```python
from build123d import *

# Parameters (mm, degrees)
BOSS_EXTRUDE1_DEPTH = 11.35
CUT_EXTRUDE1_DEPTH  = 6.35
BOSS_EXTRUDE2_DEPTH = 47
CUT_EXTRUDE2_DEPTH  = 47


with BuildPart() as part:
    # Sketch1 → Boss-Extrude1 (new body, symmetric)
    with BuildSketch(Plane.XY):
        Polygon((0, 0), (0, 47), (-17, 47), (-47, 17), (-47, 0), align=None)
    extrude(amount=BOSS_EXTRUDE1_DEPTH, both=True)

    # Sketch2 → Cut-Extrude1 (cut, symmetric)
    with BuildSketch(Plane.XY):
        Polygon((-47, 17), (-47, 2), (-2, 2), (-2, 47), (-17, 47), align=None)
    extrude(amount=CUT_EXTRUDE1_DEPTH, both=True, mode=Mode.SUBTRACT)

    # Sketch3 → Boss-Extrude2 (add)
    with BuildSketch(Plane(origin=(0, 0, -11.35), x_dir=(-1, 0, 0), z_dir=(0, 0, -1))):
        Polygon((0, 0), (0, 2), (0, 14.7), (0, 16.7), (47, 16.7), (47, 14.7), (2, 14.7), (2, 2), (47, 2), (47, 0), align=None)
    extrude(amount=BOSS_EXTRUDE2_DEPTH)

    # Sketch4 → Cut-Extrude2 (cut)
    with BuildSketch(Plane(origin=(0, 16.7, 0), x_dir=(1, 0, 0), z_dir=(0, 1, 0))):
        Polygon((-17, 58.35), (-47, 28.35), (-47, 58.35), align=None)
    extrude(amount=-CUT_EXTRUDE2_DEPTH, mode=Mode.SUBTRACT)


solid = part.part
```
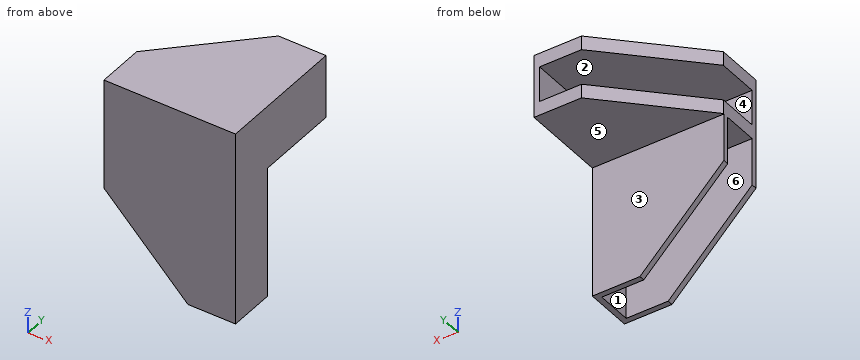
Model file for the job. Use its own axes, mm. Face numbers are marked on the shaded views. A direction names the side the tool comes from. Give positions to 0.01 mm unless a question says otherwise; leave off trailing zeros. Order: outer loops, then holes, each group sorted by start corner. A loop starts at its lowest first (then second) coordinate and runs counter-clockwise, first axis right, second up.
1) Saw through at D-D, the plane y = 6.5. Write the cut outline in (x, z), then the cut area to 3 significant figures.
2) Wall check: probe 1 along Y at (x, z) = (-7, -42); probe 2 along Z at (x, y) = (-26, 30); probe 3 along X at (y, z) = (9, -50). Give the ranges that are in metal, low to high.
3) Saw through at C-C, the plane x = -37. Write the cut outline in (y, z), then the cut area to 3 significant figures.
4) Mould opens along Z. For the marked faces 4, 5 and 6 say: +Z half, -Z half, draft (parallel to the pull), parting line (faces both ways), or undercut.
5) Pin check, flat tips, straight feed: pin 1 (22.5 mm diameter, centred on x = -17, y = 29.5, fed in from -Z); pin 2 (4 mm diameter, centred on x = -21, z = 0.5, fed in from +Y); pin 3 (2 mm diameter, centred on y = 18, z = -26, fed in from +X); pin 4 (10 mm diameter, centred on y = 7.5, z = -29.5, fed in from -X). Stop position of each tip, or through.
6) Saw through at A-A, the plane z = -20. Write the cut outline in (x, y).
7) 3-axis set-ups, long thin cutter, end or side, ignore diameter. For the marked faces 1, 2 and 3: which of +Z, -Z, +X, -X, +Y, -Y reach the whole face in a straight line?
8) Saw through at B-B, the plane y = 42. Write the cut outline in (x, z), then the cut area to 3 significant figures.
Computed:
1. outline: (-47, -11.35) - (-2, -11.35) - (-2, -58.35) - (0, -58.35) - (0, 11.35) - (-47, 11.35) - (-47, 6.35) - (-2, 6.35) - (-2, -6.35) - (-47, -6.35) - close
1. area: 589 mm2
2. probe 1: y = 0 to 2, 14.7 to 16.7
2. probe 2: z = -11.35 to -6.35, 6.35 to 11.35
2. probe 3: x = -2 to 0
3. outline: (0, -38.35) - (2, -38.35) - (2, -11.35) - (14.7, -11.35) - (14.7, -38.35) - (16.7, -38.35) - (16.7, -11.35) - (27, -11.35) - (27, -6.35) - (2, -6.35) - (2, 6.35) - (27, 6.35) - (27, 11.35) - (0, 11.35) - close
3. area: 403 mm2
4. face 4: undercut
4. face 5: -Z half
4. face 6: draft
5. pin 1: stops at z = -11.35
5. pin 2: stops at y = 2
5. pin 3: passes through
5. pin 4: stops at x = -2
6. outline: (-47, 0) - (0, 0) - (0, 16.7) - (-47, 16.7) - (-47, 14.7) - (-2, 14.7) - (-2, 2) - (-47, 2) - close
7. face 1: -Z, -X
7. face 2: -X, +Y
7. face 3: -Z, +X, -X, +Y
8. outline: (-22, -11.35) - (0, -11.35) - (0, 11.35) - (-22, 11.35) - (-22, 6.35) - (-2, 6.35) - (-2, -6.35) - (-22, -6.35) - close
8. area: 245 mm2
